Here's the drawing with two shaded views (mm, measured from the low corner). I have some questions. A direction names the side the tool comes from. Coordinates: 2 decimals unless noted, no trailing zeros. Order: outer loops, then holes, each group sorted by start corner. A loop starts at its lowest first (then second) coordinate and runs counter-clockwise, first axis right, second up. Notation, with made-up numbers: (28.5, -35.75) -> (67.5, -35.75) arc R14 ccw to (67.5, -8.75) -> close; hole circle Ø3 at (85.25, 8). An arc over 180 degrees is marked (long way). Return JSON: item names as keys, results as strings. Group by question number.
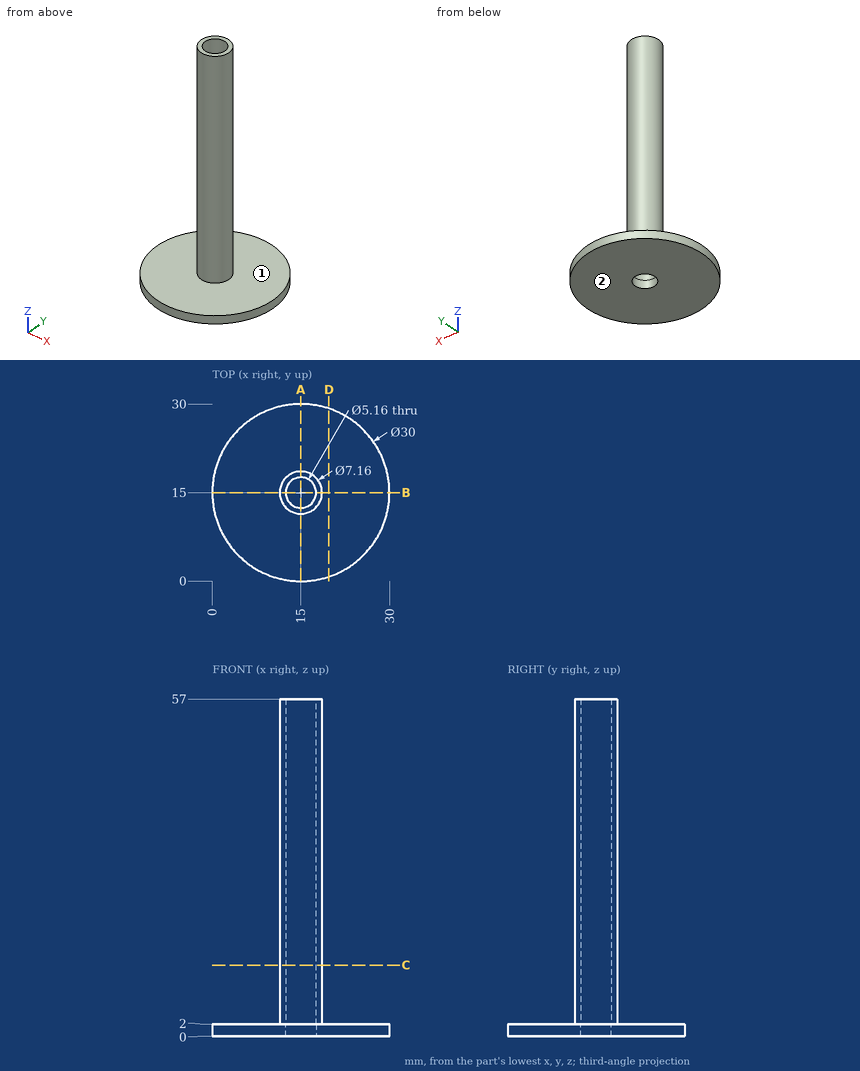
Q1. I'm going to push flat-ended pins straight in: pin 1 Ø9 at (x, y) = (8, 10.5) entering from +Z; pin 2 Ø4 at (y, z) = (16, 30) entering from +X; pin 3 Ø4 at (x, z) = (12, 27.5) entering from +Y. Where does each tip first touch, or does it pass through?
Q2. I want a section at A-A on x = 15. Please give me the cut outline in (y, z), and give its area (3 significant figures).
Q3. I want a section at D-D on x = 19.75. Please give me the cut outline in (y, z), and give its area (3 significant figures).
Q4. I need wall thicknesses on line 1 along Y through (x, z) = (15, 39.5); line 2 along Z through (x, y) = (21, 5); line 3 along Y through (x, z) = (15, 0.7). Which ranges of each line are inside material? Lowest first, please. Write a range as from..to.
Q5. On a 3-axis mill with a long thin cutter (end or side, diameter ignored), from which of +Z, -Z, +X, -X, +Y, -Y can I reach the whole of each face in a straight line? I mean the marked faces 1 and 2. Say none if no direction works.
Q6. I want a section at C-C on z = 12. Please give me the cut outline in (x, y).
Response values:
{
 "1": {"pin 1": "stops at z = 2", "pin 2": "stops at x = 18.58", "pin 3": "stops at y = 18.44"},
 "2": {"outline": "(0, 0) -> (12.42, 0) -> (12.42, 57) -> (11.42, 57) -> (11.42, 2) -> (0, 2) -> close; (17.58, 0) -> (30, 0) -> (30, 2) -> (18.58, 2) -> (18.58, 57) -> (17.58, 57) -> close", "area": "160 mm²"},
 "3": {"outline": "(0.77, 0) -> (29.23, 0) -> (29.23, 2) -> (0.77, 2) -> close", "area": "56.9 mm²"},
 "4": {"line 1": "y = 11.42..12.42, 17.58..18.58", "line 2": "z = 0..2", "line 3": "y = 0..12.42, 17.58..30"},
 "5": {"face 1": "+Z", "face 2": "-Z, +X, -X, +Y, -Y"},
 "6": {"outline": "circle Ø7.16 at (15, 15); hole circle Ø5.16 at (15, 15)"}
}
